```python
from build123d import *

# Parameters (mm, degrees)
SKETCH1_W           = 20
SKETCH1_H           = 8
SKETCH1_W_2         = 18.4
SKETCH1_H_2         = 6.4
BOSS_EXTRUDE1_DEPTH = 10
SKETCH3_W           = 18.4
SKETCH3_H           = 6.4
BOSS_EXTRUDE2_DEPTH = 0.8
CUT_EXTRUDE1_REACH  = 10
SKETCH2_W           = 3
SKETCH2_H           = 8


with BuildPart() as part:
    # Sketch1 → Boss-Extrude1 (new body)
    with BuildSketch(Plane(origin=(0, 0, 0), x_dir=(1, 0, 0), z_dir=(0, 1, 0))):
        Rectangle(SKETCH1_W, SKETCH1_H)
        Rectangle(SKETCH1_W_2, SKETCH1_H_2, mode=Mode.SUBTRACT)
    extrude(amount=BOSS_EXTRUDE1_DEPTH)

    # Sketch3 → Boss-Extrude2 (add)
    with BuildSketch(Plane(origin=(0, 0, 0), x_dir=(1, 0, 0), z_dir=(0, 1, 0))):
        Rectangle(SKETCH3_W, SKETCH3_H)
    extrude(amount=BOSS_EXTRUDE2_DEPTH)

    # Sketch2 → Cut-Extrude1 (cut, up to next)
    with BuildSketch(Plane.XY.offset(-4), mode=Mode.PRIVATE) as cut_extrude1_sk1:
        with Locations((0, 6)):
            Rectangle(SKETCH2_W, SKETCH2_H)
    cut_extrude1_tool1 = extrude(cut_extrude1_sk1.sketch, amount=CUT_EXTRUDE1_REACH, mode=Mode.PRIVATE) & part.part
    add(cut_extrude1_tool1.solids().sort_by_distance((0, 6, -4))[0], mode=Mode.SUBTRACT)


solid = part.part
```
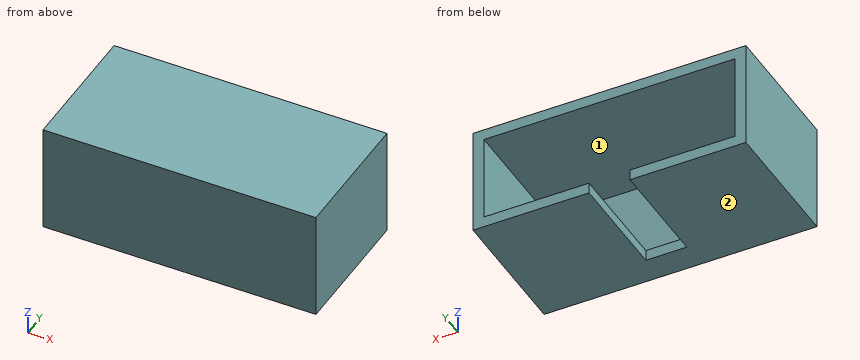
Input: part model. Units: mm. Frame: model coordinates. Face numbers are marked on the shaded views. A direction names the side the tool comes from. Coordinates: 2 decimals unless noted, no trailing zeros. Write each loop counter-clockwise with the first axis right and the second up, starting at its lowest first coordinate (ties: lowest second). Pieces come first, ordered by that corner, then holes.
1) Material intervals for line 1 along Z through (x, y) = (-8.75, 1.25); line 2 along X through (y, z) = (6.25, 2.5); line 3 along Y through (x, z) = (1.5, -3), sorted ascending.
2) Section A-A on y = 1.25. Output: boundary loops of the cut face in (x, z).
3) Section C-C on y = 3.25. Output: boundary loops of the cut face in (x, z).
4) Section D-D on z = 2.5. Output: boundary loops of the cut face in (x, y).
5) Section B-B on x = -0.5. Output: boundary loops of the cut face in (y, z).
6) Set-up query: the marked faces 1 and 2. Return all of +Z, -Z, +X, -X, +Y, -Y with unobstructed straight access to the full face (end or side cutting, diameter ignored); none if empty.
7) Pin query (flat end, axial travel): pin 1 Ø1 at (x, z) = (-5.5, -0.5) entering from +Y; pin 2 Ø0.9 at (x, z) = (-0.5, -3.5) entering from +Y. Return the tip coordinate at first contact, or that it passes through.
Check result:
1. line 1: z = -4 to -3.2, 3.2 to 4
1. line 2: x = -10 to -9.2, 9.2 to 10
1. line 3: y = 0 to 0.8
2. outline: (-10, -4) - (10, -4) - (10, 4) - (-10, 4) - close; hole (-9.2, -3.2) - (9.2, -3.2) - (9.2, 3.2) - (-9.2, 3.2) - close
3. outline: (-10, -4) - (-1.5, -4) - (-1.5, -3.2) - (-9.2, -3.2) - (-9.2, 3.2) - (9.2, 3.2) - (9.2, -3.2) - (1.5, -3.2) - (1.5, -4) - (10, -4) - (10, 4) - (-10, 4) - close
4. outline: (-10, 0) - (10, 0) - (10, 10) - (9.2, 10) - (9.2, 0.8) - (-9.2, 0.8) - (-9.2, 10) - (-10, 10) - close
5. outline: (0, -4) - (2, -4) - (2, -3.2) - (0.8, -3.2) - (0.8, 3.2) - (10, 3.2) - (10, 4) - (0, 4) - close
6. face 1: +Y
6. face 2: -Z, +X, -X, +Y, -Y
7. pin 1: stops at y = 0.8
7. pin 2: stops at y = 2
